```python
from build123d import *

# Parameters (mm, degrees)
F1_DEPTH = 10.16
F2_R     = 3
F4_DEPTH = 1
F6_DEPTH = 11.16
F8_DEPTH = 11.16


with BuildPart() as f1:
    # F0 (on Top) → F1 (new body)
    with BuildSketch(Plane.XY):
        with BuildLine():
            Line((2.4892, 8.382), (2.4892, 6.35))
            Line((2.4892, 6.35), (0.5, 6.35))
            ThreePointArc((0.5, 6.35), (0.4999030778, 6.340155572), (0.499612349, 6.3303149606))
            ThreePointArc((0.499612349, 6.3303149606), (4.4901280605, 4.4901280605), (6.3303149606, 0.499612349))
            ThreePointArc((6.3303149606, 0.499612349), (6.340155572, 0.4999030778), (6.35, 0.5))
            Line((6.35, 0.5), (6.35, 2.4892))
            Line((6.35, 2.4892), (8.382, 2.4892))
            Line((8.382, 2.4892), (8.382, -2.4892))
            Line((8.382, -2.4892), (6.35, -2.4892))
            Line((6.35, -2.4892), (6.35, -0.5))
            ThreePointArc((6.35, -0.5), (6.340155572, -0.4999030778), (6.3303149606, -0.499612349))
            ThreePointArc((6.3303149606, -0.499612349), (5.9570857831, -2.1990063604), (5.1366242038, -3.733308424))
            Line((5.1366242038, -3.733308424), (6.35, -4.6151923037))
            ThreePointArc((6.35, -4.6151923037), (6.5628814967, -4.3070972197), (6.760827121, -3.9892))
            Line((6.760827121, -3.9892), (9.882, -3.9892))
            Line((9.882, -3.9892), (9.882, 3.9892))
            Line((9.882, 3.9892), (6.760827121, 3.9892))
            ThreePointArc((6.760827121, 3.9892), (5.5507882323, 5.5507882323), (3.9892, 6.760827121))
            Line((3.9892, 6.760827121), (3.9892, 9.882))
            Line((3.9892, 9.882), (-3.9892, 9.882))
            Line((-3.9892, 9.882), (-3.9892, 6.760827121))
            ThreePointArc((-3.9892, 6.760827121), (-5.5507882323, 5.5507882323), (-6.760827121, 3.9892))
            Line((-6.760827121, 3.9892), (-9.882, 3.9892))
            Line((-9.882, 3.9892), (-9.882, -3.9892))
            Line((-9.882, -3.9892), (-6.760827121, -3.9892))
            ThreePointArc((-6.760827121, -3.9892), (-6.5628814967, -4.3070972197), (-6.35, -4.6151923037))
            Line((-6.35, -4.6151923037), (-5.1366242038, -3.733308424))
            ThreePointArc((-5.1366242038, -3.733308424), (-5.3088277076, -3.4840850121), (-5.4689493272, -3.2269324841))
            ThreePointArc((-5.4689493272, -3.2269324841), (-6.0551819306, -1.9123994841), (-6.3303149606, -0.499612349))
            ThreePointArc((-6.3303149606, -0.499612349), (-6.340155572, -0.4999030778), (-6.35, -0.5))
            Line((-6.35, -0.5), (-6.35, -2.4892))
            Line((-6.35, -2.4892), (-8.382, -2.4892))
            Line((-8.382, -2.4892), (-8.382, 2.4892))
            Line((-8.382, 2.4892), (-6.35, 2.4892))
            Line((-6.35, 2.4892), (-6.35, 0.5))
            ThreePointArc((-6.35, 0.5), (-6.340155572, 0.4999030778), (-6.3303149606, 0.499612349))
            ThreePointArc((-6.3303149606, 0.499612349), (-4.4901280605, 4.4901280605), (-0.499612349, 6.3303149606))
            ThreePointArc((-0.499612349, 6.3303149606), (-0.4999030778, 6.340155572), (-0.5, 6.35))
            Line((-0.5, 6.35), (-2.4892, 6.35))
            Line((-2.4892, 6.35), (-2.4892, 8.382))
            Line((-2.4892, 8.382), (2.4892, 8.382))
        make_face()
    extrude(amount=F1_DEPTH)

    # F2
    f2_edges = [f1.edges().sort_by_distance(p)[0] for p in [
        (-3.9892, 9.882, 5.08),
        (3.9892, 9.882, 5.08),
        (-9.882, 3.9892, 5.08),
        (-9.882, -3.9892, 5.08),
        (9.882, 3.9892, 5.08),
        (9.882, -3.9892, 5.08),
    ]]
    fillet(f2_edges, radius=F2_R)

    # F3 (on face) → F4 (join)
    with BuildSketch(Plane.XY.offset(10.16)):
        with BuildLine():
            ThreePointArc((-3.9892, 6.760827121), (-5.5507882323, 5.5507882323), (-6.760827121, 3.9892))
            Line((-6.760827121, 3.9892), (-6.882, 3.9892))
            ThreePointArc((-6.882, 3.9892), (-9.0033203436, 3.1105203436), (-9.882, 0.9892))
            Line((-9.882, 0.9892), (-9.882, -0.9892))
            ThreePointArc((-9.882, -0.9892), (-9.0033203436, -3.1105203436), (-6.882, -3.9892))
            Line((-6.882, -3.9892), (-6.760827121, -3.9892))
            ThreePointArc((-6.760827121, -3.9892), (-6.5628814967, -4.3070972197), (-6.35, -4.6151923037))
            Line((-6.35, -4.6151923037), (-5.1366242038, -3.733308424))
            ThreePointArc((-5.1366242038, -3.733308424), (-5.9570857831, -2.1990063604), (-6.3303149606, -0.499612349))
            ThreePointArc((-6.3303149606, -0.499612349), (-6.340155572, -0.4999030778), (-6.35, -0.5))
            Line((-6.35, -0.5), (-6.35, -2.4892))
            Line((-6.35, -2.4892), (-8.382, -2.4892))
            Line((-8.382, -2.4892), (-8.382, 2.4892))
            Line((-8.382, 2.4892), (-6.35, 2.4892))
            Line((-6.35, 2.4892), (-6.35, 0.5))
            ThreePointArc((-6.35, 0.5), (-6.340155572, 0.4999030778), (-6.3303149606, 0.499612349))
            ThreePointArc((-6.3303149606, 0.499612349), (-4.4901280605, 4.4901280605), (-0.499612349, 6.3303149606))
            ThreePointArc((-0.499612349, 6.3303149606), (-0.4999030778, 6.340155572), (-0.5, 6.35))
            Line((-0.5, 6.35), (-2.4892, 6.35))
            Line((-2.4892, 6.35), (-2.4892, 8.382))
            Line((-2.4892, 8.382), (2.4892, 8.382))
            Line((2.4892, 8.382), (2.4892, 6.35))
            Line((2.4892, 6.35), (0.5, 6.35))
            ThreePointArc((0.5, 6.35), (0.4999030778, 6.340155572), (0.499612349, 6.3303149606))
            ThreePointArc((0.499612349, 6.3303149606), (4.4901280605, 4.4901280605), (6.3303149606, 0.499612349))
            ThreePointArc((6.3303149606, 0.499612349), (6.340155572, 0.4999030778), (6.35, 0.5))
            Line((6.35, 0.5), (6.35, 2.4892))
            Line((6.35, 2.4892), (8.382, 2.4892))
            Line((8.382, 2.4892), (8.382, -2.4892))
            Line((8.382, -2.4892), (6.35, -2.4892))
            Line((6.35, -2.4892), (6.35, -0.5))
            ThreePointArc((6.35, -0.5), (6.340155572, -0.4999030778), (6.3303149606, -0.499612349))
            ThreePointArc((6.3303149606, -0.499612349), (5.9570857831, -2.1990063604), (5.1366242038, -3.733308424))
            Line((5.1366242038, -3.733308424), (6.35, -4.6151923037))
            ThreePointArc((6.35, -4.6151923037), (6.5628814967, -4.3070972197), (6.760827121, -3.9892))
            Line((6.760827121, -3.9892), (6.882, -3.9892))
            ThreePointArc((6.882, -3.9892), (9.0033203436, -3.1105203436), (9.882, -0.9892))
            Line((9.882, -0.9892), (9.882, 0.9892))
            ThreePointArc((9.882, 0.9892), (9.0033203436, 3.1105203436), (6.882, 3.9892))
            Line((6.882, 3.9892), (6.760827121, 3.9892))
            ThreePointArc((6.760827121, 3.9892), (5.5507882323, 5.5507882323), (3.9892, 6.760827121))
            Line((3.9892, 6.760827121), (3.9892, 6.882))
            ThreePointArc((3.9892, 6.882), (3.1105203436, 9.0033203436), (0.9892, 9.882))
            Line((0.9892, 9.882), (-0.9892, 9.882))
            ThreePointArc((-0.9892, 9.882), (-3.1105203436, 9.0033203436), (-3.9892, 6.882))
            Line((-3.9892, 6.882), (-3.9892, 6.760827121))
        make_face()
        with BuildLine():
            ThreePointArc((-6.35, -0.5), (-6.340155572, -0.4999030778), (-6.3303149606, -0.499612349))
            ThreePointArc((-6.3303149606, -0.499612349), (-6.35, 0), (-6.3303149606, 0.499612349))
            ThreePointArc((-6.3303149606, 0.499612349), (-6.340155572, 0.4999030778), (-6.35, 0.5))
            Line((-6.35, 0.5), (-6.35, 2.4892))
            Line((-6.35, 2.4892), (-8.382, 2.4892))
            Line((-8.382, 2.4892), (-8.382, -2.4892))
            Line((-8.382, -2.4892), (-6.35, -2.4892))
            Line((-6.35, -2.4892), (-6.35, -0.5))
        make_face()
        with BuildLine():
            ThreePointArc((-0.5, 6.35), (-0.4999030778, 6.340155572), (-0.499612349, 6.3303149606))
            ThreePointArc((-0.499612349, 6.3303149606), (-0.25, 6.3450768317), (0, 6.35))
            ThreePointArc((0, 6.35), (0.25, 6.3450768317), (0.499612349, 6.3303149606))
            ThreePointArc((0.499612349, 6.3303149606), (0.4999030778, 6.340155572), (0.5, 6.35))
            Line((0.5, 6.35), (2.4892, 6.35))
            Line((2.4892, 6.35), (2.4892, 8.382))
            Line((2.4892, 8.382), (-2.4892, 8.382))
            Line((-2.4892, 8.382), (-2.4892, 6.35))
            Line((-2.4892, 6.35), (-0.5, 6.35))
        make_face()
        with BuildLine():
            ThreePointArc((6.35, 0.5), (6.340155572, 0.4999030778), (6.3303149606, 0.499612349))
            ThreePointArc((6.3303149606, 0.499612349), (6.3450768317, 0.25), (6.35, 0))
            Line((6.35, 0), (6.35, -0.5))
            Line((6.35, -0.5), (6.35, -2.4892))
            Line((6.35, -2.4892), (8.382, -2.4892))
            Line((8.382, -2.4892), (8.382, 2.4892))
            Line((8.382, 2.4892), (6.35, 2.4892))
            Line((6.35, 2.4892), (6.35, 0.5))
        make_face()
    extrude(amount=F4_DEPTH)

    # F5 (on face) → F6 (join, through all)
    with BuildSketch(Plane(origin=(0, 0, 0), x_dir=(1, 0, 0), z_dir=(0, 0, -1))):
        with BuildLine():
            ThreePointArc((3.9892, -6.882), (3.3907514875, -8.6799294905), (1.8341663648, -9.7605468282))
            ThreePointArc((1.8341663648, -9.7605468282), (7.0225508414, -7.0225508414), (9.7605468282, -1.8341663648))
            ThreePointArc((9.7605468282, -1.8341663648), (8.6799294905, -3.3907514875), (6.882, -3.9892))
            Line((6.882, -3.9892), (6.760827121, -3.9892))
            ThreePointArc((6.760827121, -3.9892), (5.5507882323, -5.5507882323), (3.9892, -6.760827121))
            Line((3.9892, -6.760827121), (3.9892, -6.882))
        make_face()
        with BuildLine():
            ThreePointArc((6.882, 3.9892), (8.6799294905, 3.3907514875), (9.7605468282, 1.8341663648))
            ThreePointArc((9.7605468282, 1.8341663648), (9.1196479712, 3.9324879556), (8.0336694496, 5.8388865219))
            Line((8.0336694496, 5.8388865219), (6.35, 4.6151923037))
            ThreePointArc((6.35, 4.6151923037), (6.5628814967, 4.3070972197), (6.760827121, 3.9892))
            Line((6.760827121, 3.9892), (6.882, 3.9892))
        make_face()
        with BuildLine():
            ThreePointArc((-8.0336694496, 5.8388865219), (-9.1196479712, 3.9324879556), (-9.7605468282, 1.8341663648))
            ThreePointArc((-9.7605468282, 1.8341663648), (-8.6799294905, 3.3907514875), (-6.882, 3.9892))
            Line((-6.882, 3.9892), (-6.760827121, 3.9892))
            ThreePointArc((-6.760827121, 3.9892), (-6.5628814967, 4.3070972197), (-6.35, 4.6151923037))
            Line((-6.35, 4.6151923037), (-8.0336694496, 5.8388865219))
        make_face()
        with BuildLine():
            Line((-3.9892, -6.882), (-3.9892, -6.760827121))
            ThreePointArc((-3.9892, -6.760827121), (-5.5507882323, -5.5507882323), (-6.760827121, -3.9892))
            Line((-6.760827121, -3.9892), (-6.882, -3.9892))
            ThreePointArc((-6.882, -3.9892), (-8.6799294905, -3.3907514875), (-9.7605468282, -1.8341663648))
            ThreePointArc((-9.7605468282, -1.8341663648), (-7.0225508414, -7.0225508414), (-1.8341663648, -9.7605468282))
            ThreePointArc((-1.8341663648, -9.7605468282), (-3.3907514875, -8.6799294905), (-3.9892, -6.882))
        make_face()
    extrude(amount=-F6_DEPTH)

    # F7 (on face) → F8 (join, through all)
    with BuildSketch(Plane(origin=(0, 0, 0), x_dir=(1, 0, 0), z_dir=(0, 0, -1))):
        with BuildLine():
            Line((-7.8282044814, 5.6895541849), (-8.2391344177, 5.9882188588))
            ThreePointArc((-8.2391344177, 5.9882188588), (0, -10.1853866424), (8.2391344177, 5.9882188588))
            Line((8.2391344177, 5.9882188588), (7.8282044814, 5.6895541849))
            ThreePointArc((7.8282044814, 5.6895541849), (0, -9.6773866424), (-7.8282044814, 5.6895541849))
        make_face()
    extrude(amount=-F8_DEPTH)


solid = f1.part
```
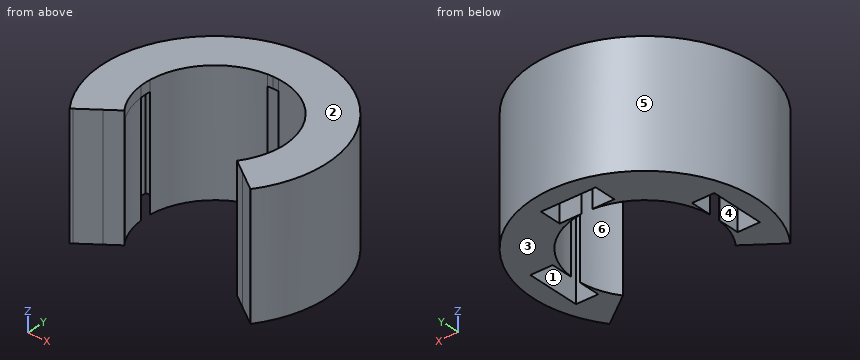
Build history of the part. All positions in model axes, mm. Face numbers are marked on the shaded views. A direction names the side the tool comes from. Coordinates: 2 decimals unless noted, no trailing zeros. Write each loop counter-clockwise with the first axis right and the second up, starting at its lowest first coordinate (ties: lowest second). Pieces come first, ordered by that corner, then holes.
1. Band-saw the part on D-D, the plane x = 7.25. Give the cut face in (y, z), and give its area (3 significant figures).
Answer block:
outline: (-5.27, 0) - (-2.49, 0) - (-2.49, 10.16) - (2.49, 10.16) - (2.49, 0) - (7.15, 0) - (7.15, 11.16) - (-5.27, 11.16) - close
area: 88.1 mm2
2. 3-axis set-ups, long thin cutter, end or side, ignore diameter. For the marked faces 1 and 2: which of +Z, -Z, +X, -X, +Y, -Y reach the whole face in a straight line?
Answer block:
face 1: -Z
face 2: +Z, +X, -X, +Y, -Y
3. Pull direction Y, two halves, no side cores. Call the marked faces 3, 4, 5 and 6: released by +Y, released by -Y, zero draft, split by the parting line, or undercut.
Answer block:
face 3: zero draft
face 4: undercut
face 5: split by the parting line
face 6: undercut
4. Drill centre lines: probe 1 along X at (y, z) = (-3, 6.5); probe 2 along X at (y, z) = (8, 5); probe 3 along Z at (x, y) = (1.25, 6.5). Where is each one in solid material? Low to high.
Answer block:
probe 1: x = -9.73 to -5.6, 5.6 to 9.73
probe 2: x = -6.3 to -2.49, 2.49 to 6.3
probe 3: z = 10.16 to 11.16
5. Band-saw the part on C-C, the plane y = 7. Give the cut face in (x, z), and give its area (3 significant figures).
Answer block:
outline: (-7.4, 0) - (-2.49, 0) - (-2.49, 10.16) - (2.49, 10.16) - (2.49, 0) - (7.4, 0) - (7.4, 11.16) - (-7.4, 11.16) - close
area: 115 mm2
6. Band-saw the part on A-A, the plane y = 5. Give the cut face in (x, z).
Answer block:
outline: (-8.87, 0) - (-3.91, 0) - (-3.91, 11.16) - (-8.87, 11.16) - close; (3.91, 0) - (8.87, 0) - (8.87, 11.16) - (3.91, 11.16) - close
7. Drop flat-ended pins along their axis: pin 1 (5 mm diameter, centred on y = -1, z = 1.5, fed in from -X); pin 2 (1.5 mm diameter, centred on x = 8, z = 6, fed in from +Y); pin 3 (1 mm diameter, centred on x = -7, z = 7.5, fed in from -Y); pin 4 (0.6 mm diameter, centred on x = -1.5, z = 6.5, fed in from +Y). Give the stop position or say it passes through.
Answer block:
pin 1: stops at x = -10.19
pin 2: stops at y = 7.15
pin 3: stops at y = -5.45
pin 4: stops at y = 10.11
